The listing builds one solid part. Answer for the finished solid, in the listing's coordinates (mm). Round coordinates to 2 decimals unless told otherwise and drop trailing zeros. Write each loop counter-clockwise with the first axis right and the second up, starting at its lowest first coordinate (ties: lowest second). Pieces come first, ordered by that corner, then holes.
Item 1: Find section B-B on x = 27. Give the vertices of the cut face in (y, z), then the cut area to 3 significant figures.
Item 2: For a pull along X with two mould halves and no side action, classify faces 1 (the face through (198, 15.18, -324)), 2 (the face through (-104.123, 7.977, -298.737)), 3 (the face through (221, 0, -232)) as +X half, -X half, draft (parallel to the pull), parting line (faces both ways), or undercut.
Item 3: Find section C-C on z = -410. Give the vertices of the cut face in (x, y).
Item 4: Each of these flat-tipped pins is pushed along its axis until it touches: pin 1 (5 mm diameter, centred on x = 417.675, z = -344.325, fed in from -Y); pin 2 (1 mm diameter, centred on x = 305, y = 14.5, fed in from -Z); pin 3 (3 mm diameter, centred on y = 5.5, z = -167.5, fed in from +X); pin 4 (2.5 mm diameter, centred on x = 417.675, z = -59.325, fed in from +Y). Where does it stop, or does it pass through?
Item 5: Find the intervals of material crossed by probe 1 along X at (y, z) = (3, -71); probe 2 along Y at (x, z) = (19, -61); probe 3 along X at (y, z) = (8, -343), in increasing order.
Item 6: Find section A-A on y = 12.5. Give the number of separate pieces and of enclosed holes in the cut face, then the cut area to 3 significant figures.
```python
from build123d import *

# Parameters (mm, degrees)
SKETCH1_R           = 328.6125
BOSS_EXTRUDE1_DEPTH = 16.1798
SKETCH3_R           = 2.25
CUT_EXTRUDE1_DEPTH  = 780.013065513
SKETCH4_W           = 42.25
SKETCH4_H           = 42.25
CUT_EXTRUDE2_DEPTH  = 1
SKETCH5_R           = 3.75
CUT_EXTRUDE3_DEPTH  = 7.5


with BuildPart() as part:
    # Sketch1 → Boss-Extrude1 (new body)
    with BuildSketch(Plane(origin=(0, 0, 0), x_dir=(1, 0, 0), z_dir=(0, 1, 0))):
        with Locations(Location((216.675, 227.5, 0), (0, 0, 270))):
            Circle(SKETCH1_R)
    extrude(amount=BOSS_EXTRUDE1_DEPTH)

    # Sketch3 → Cut-Extrude1 (cut, through all)
    with BuildSketch(Plane(origin=(0, 16.1798, 0), x_dir=(1, 0, 0), z_dir=(0, 1, 0))):
        with Locations(Location((322.675, 439.325, 0), (0, 0, 270))):
            Circle(SKETCH3_R)
        with Locations(Location((307.675, 439.325, 0), (0, 0, 270))):
            Circle(SKETCH3_R)
        with Locations(Location((110.675, 439.325, 0), (0, 0, 270))):
            Circle(SKETCH3_R)
        with Locations(Location((125.675, 439.325, 0), (0, 0, 270))):
            Circle(SKETCH3_R)
        with Locations(Location((183.215, 375.2, 0), (0, 0, 270))):
            Circle(SKETCH3_R)
        with Locations(Location((213.215, 375.2, 0), (0, 0, 270))):
            Circle(SKETCH3_R)
        with Locations(Location((15.675, 329.325, 0), (0, 0, 270))):
            Circle(SKETCH3_R)
        with Locations(Location((15.675, 344.325, 0), (0, 0, 270))):
            Circle(SKETCH3_R)
        with Locations(Location((417.675, 329.325, 0), (0, 0, 270))):
            Circle(SKETCH3_R)
        with Locations(Location((417.675, 344.325, 0), (0, 0, 270))):
            Circle(SKETCH3_R)
        with Locations(Location((417.675, 59.325, 0), (0, 0, 270))):
            Circle(SKETCH3_R)
        with Locations(Location((417.675, 74.325, 0), (0, 0, 270))):
            Circle(SKETCH3_R)
        with Locations(Location((15.675, 59.325, 0), (0, 0, 270))):
            Circle(SKETCH3_R)
        with Locations(Location((15.675, 74.325, 0), (0, 0, 270))):
            Circle(SKETCH3_R)
        with Locations(Location((303.215, 378.325, 0), (0, 0, 270))):
            Circle(SKETCH3_R)
        with Locations(Location((273.215, 378.325, 0), (0, 0, 270))):
            Circle(SKETCH3_R)
        with Locations(Location((123.215, 378.325, 0), (0, 0, 270))):
            Circle(SKETCH3_R)
        with Locations(Location((93.215, 378.325, 0), (0, 0, 270))):
            Circle(SKETCH3_R)
    extrude(amount=-CUT_EXTRUDE1_DEPTH, mode=Mode.SUBTRACT)

    # Sketch4 → Cut-Extrude2 (cut)
    with BuildSketch(Plane(origin=(0, 16.1798, 0), x_dir=(1, 0, 0), z_dir=(0, 1, 0))):
        with Locations((198.125, 323.875)):
            Rectangle(SKETCH4_W, SKETCH4_H)
    extrude(amount=-CUT_EXTRUDE2_DEPTH, mode=Mode.SUBTRACT)

    # Sketch5 → Cut-Extrude3 (cut)
    with BuildSketch(Plane.XZ):
        with Locations(Location((15.675, -59.325, 0), (0, 0, 270))):
            Circle(SKETCH5_R)
        with Locations(Location((15.675, -74.325, 0), (0, 0, 270))):
            Circle(SKETCH5_R)
        with Locations(Location((15.675, -344.325, 0), (0, 0, 270))):
            Circle(SKETCH5_R)
        with Locations(Location((15.675, -329.325, 0), (0, 0, 270))):
            Circle(SKETCH5_R)
        with Locations(Location((93.215, -378.325, 0), (0, 0, 270))):
            Circle(SKETCH5_R)
        with Locations(Location((123.215, -378.325, 0), (0, 0, 270))):
            Circle(SKETCH5_R)
        with Locations(Location((183.215, -375.2, 0), (0, 0, 270))):
            Circle(SKETCH5_R)
        with Locations(Location((213.215, -375.2, 0), (0, 0, 270))):
            Circle(SKETCH5_R)
        with Locations(Location((273.215, -378.325, 0), (0, 0, 270))):
            Circle(SKETCH5_R)
        with Locations(Location((125.675, -439.325, 0), (0, 0, 270))):
            Circle(SKETCH5_R)
        with Locations(Location((110.675, -439.325, 0), (0, 0, 270))):
            Circle(SKETCH5_R)
        with Locations(Location((303.215, -378.325, 0), (0, 0, 270))):
            Circle(SKETCH5_R)
        with Locations(Location((307.675, -439.325, 0), (0, 0, 270))):
            Circle(SKETCH5_R)
        with Locations(Location((322.675, -439.325, 0), (0, 0, 270))):
            Circle(SKETCH5_R)
        with Locations(Location((417.675, -344.325, 0), (0, 0, 270))):
            Circle(SKETCH5_R)
        with Locations(Location((417.675, -329.325, 0), (0, 0, 270))):
            Circle(SKETCH5_R)
        with Locations(Location((417.675, -74.325, 0), (0, 0, 270))):
            Circle(SKETCH5_R)
        with Locations(Location((417.675, -59.325, 0), (0, 0, 270))):
            Circle(SKETCH5_R)
    extrude(amount=-CUT_EXTRUDE3_DEPTH, mode=Mode.SUBTRACT)


solid = part.part
```
Check values:
1. outline: (0, -495.85) - (16.18, -495.85) - (16.18, 40.85) - (0, 40.85) - close
1. area: 8,680 mm2
2. face 1: undercut
2. face 2: parting line
2. face 3: draft
3. outline: (-56.6, 0) - (489.95, 0) - (489.95, 16.18) - (-56.6, 16.18) - close
4. pin 1: stops at y = 7.5
4. pin 2: stops at z = -544.16
4. pin 3: stops at x = 540.04
4. pin 4: passes through
5. probe 1: x = -72.28 to 13.94, 17.41 to 415.94, 419.41 to 505.63
5. probe 2: y = 7.5 to 16.18
5. probe 3: x = -90.97 to 13.86, 17.49 to 415.86, 419.49 to 524.32
6. separate pieces: 1
6. enclosed holes: 18
6. area: 339,000 mm2
